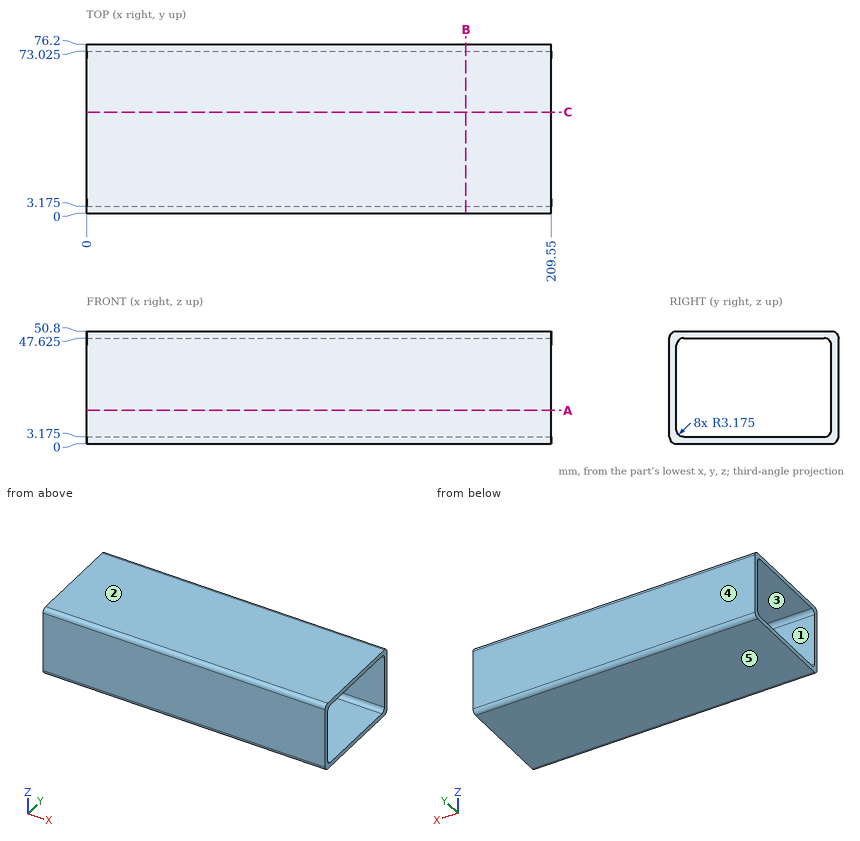
Input: dimensioned drawing with shaded views. Units: mm. Origin: part minimum x, y, z. A direction names the side the tool comes from. Round coordinates to 2 decimals unless told otherwise and drop trailing zeros. Loops run counter-clockwise (first coordinate to the right, second up) from the corner with the lowest first, then second, coordinate; pieces in that order, holes last. Notation, with made-up numbers: (30.5, 50.25) -> (58.5, 50.25) arc R23 cw to (58.5, 88.25) -> close; hole circle Ø6 at (-29, 24). An arc over 180 degrees is marked (long way). Answer as a JSON object with one key per item and string values. Group by question number.
Q1. Section query A-A (z = 15). Output: boundary loops of the cut face in (x, y) (3 decimals), plus the area to 3 significant figures.
Q2. Ray query, line 1 (Y direction, x = 17, z = 36) (3 decimals); line 2 (Z direction, x = 133, y = 42) (3 decimals); line 3 (Y direction, x = 153, z = 3). Return the intervals inside material, ascending. Write a range as from..to.
Q3. Section query C-C (y = 45.5). Output: boundary loops of the cut face in (x, z) (3 decimals).
Q4. Access query for the marked faces 1 and 2. Directions: +Z, -Z, +X, -X, +Y, -Y. A direction counts if a zero-diameter tool reaches every point of the face in a straight line with its end or side. Return the directions, or none.
Q5. Section query B-B (x = 171). Output: boundary loops of the cut face in (y, z) (3 decimals).
Q6. Mould query, pull axis Z, two halves, no side actions, for the marked faces 3, 4 and 5. Classes: pulls with the +Z half, pulls with the -Z half, needs draft (parallel to the pull), parting line crosses it, or undercut.
Completed:
{
 "1": {"outline": "(0, 0) -> (209.55, 0) -> (209.55, 3.175) -> (0, 3.175) -> close; (0, 73.025) -> (209.55, 73.025) -> (209.55, 76.2) -> (0, 76.2) -> close", "area": "1,330 mm²"},
 "2": {"line 1": "0..3.175, 73.025..76.2", "line 2": "0..3.175, 47.625..50.8", "line 3": "0..76.2"},
 "3": {"outline": "(0, 0) -> (209.55, 0) -> (209.55, 3.175) -> (0, 3.175) -> close; (0, 47.625) -> (209.55, 47.625) -> (209.55, 50.8) -> (0, 50.8) -> close"},
 "4": {"face 1": "+X, -X", "face 2": "+Z, +X, -X, +Y, -Y"},
 "5": {"outline": "(0, 3.175) arc R3.175 ccw to (3.175, 0) -> (73.025, 0) arc R3.175 ccw to (76.2, 3.175) -> (76.2, 47.625) arc R3.175 ccw to (73.025, 50.8) -> (3.175, 50.8) arc R3.175 ccw to (0, 47.625) -> close; hole (3.175, 6.35) arc R3.175 ccw to (6.35, 3.175) -> (69.85, 3.175) arc R3.175 ccw to (73.025, 6.35) -> (73.025, 44.45) arc R3.175 ccw to (69.85, 47.625) -> (6.35, 47.625) arc R3.175 ccw to (3.175, 44.45) -> close"},
 "6": {"face 3": "undercut", "face 4": "needs draft", "face 5": "pulls with the -Z half"}
}
